```python
from build123d import *

# Parameters (mm, degrees)
F1_DEPTH = 0.26


with BuildPart() as f1:
    # F0 (on Top) → F1 (new body)
    with BuildSketch(Plane.XY):
        with BuildLine():
            ThreePointArc((6.5, 0), (6.4967926424, 0.204169934), (6.4871737348, 0.4081383769))
            ThreePointArc((6.4871737348, 0.4081383769), (6.3848671297, 1.2179785448), (6.1818673559, 2.0086104634))
            ThreePointArc((6.1818673559, 2.0086104634), (5.881375841, 2.7675653952), (5.4881315158, 3.4828741674))
            ThreePointArc((5.4881315158, 3.4828741674), (5.008336078, 4.1432559334), (4.4495561885, 4.7382960782))
            ThreePointArc((4.4495561885, 4.7382960782), (3.8206041399, 5.2586104634), (3.1313988817, 5.6959934203))
            ThreePointArc((3.1313988817, 5.6959934203), (2.3928095925, 6.0435471583), (1.6164842666, 6.2957905473))
            ThreePointArc((1.6164842666, 6.2957905473), (0.8146660182, 6.4487455585), (0, 6.5))
            ThreePointArc((0, 6.5), (-0.8146660182, 6.4487455585), (-1.6164842666, 6.2957905473))
            ThreePointArc((-1.6164842666, 6.2957905473), (-2.3928095925, 6.0435471583), (-3.1313988817, 5.6959934203))
            ThreePointArc((-3.1313988817, 5.6959934203), (-3.8206041399, 5.2586104634), (-4.4495561885, 4.7382960782))
            ThreePointArc((-4.4495561885, 4.7382960782), (-5.008336078, 4.1432559334), (-5.4881315158, 3.4828741674))
            ThreePointArc((-5.4881315158, 3.4828741674), (-5.881375841, 2.7675653952), (-6.1818673559, 2.0086104634))
            ThreePointArc((-6.1818673559, 2.0086104634), (-6.3848671297, 1.2179785448), (-6.4871737348, 0.4081383769))
            ThreePointArc((-6.4871737348, 0.4081383769), (-6.4871737348, -0.4081383769), (-6.3848671297, -1.2179785448))
            ThreePointArc((-6.3848671297, -1.2179785448), (-6.1818673559, -2.0086104634), (-5.881375841, -2.7675653952))
            ThreePointArc((-5.881375841, -2.7675653952), (-5.4881315158, -3.4828741674), (-5.008336078, -4.1432559334))
            ThreePointArc((-5.008336078, -4.1432559334), (-4.4495561885, -4.7382960782), (-3.8206041399, -5.2586104634))
            ThreePointArc((-3.8206041399, -5.2586104634), (-3.1313988817, -5.6959934203), (-2.3928095925, -6.0435471583))
            ThreePointArc((-2.3928095925, -6.0435471583), (-1.6164842666, -6.2957905473), (-0.8146660182, -6.4487455585))
            ThreePointArc((-0.8146660182, -6.4487455585), (0, -6.5), (0.8146660182, -6.4487455585))
            ThreePointArc((0.8146660182, -6.4487455585), (1.6164842666, -6.2957905473), (2.3928095925, -6.0435471583))
            ThreePointArc((2.3928095925, -6.0435471583), (3.1313988817, -5.6959934203), (3.8206041399, -5.2586104634))
            ThreePointArc((3.8206041399, -5.2586104634), (4.4495561885, -4.7382960782), (5.008336078, -4.1432559334))
            ThreePointArc((5.008336078, -4.1432559334), (5.4881315158, -3.4828741674), (5.881375841, -2.7675653952))
            ThreePointArc((5.881375841, -2.7675653952), (6.1818673559, -2.0086104634), (6.3848671297, -1.2179785448))
            ThreePointArc((6.3848671297, -1.2179785448), (6.4711527699, -0.6117040366), (6.5, 0))
        make_face()
    extrude(amount=F1_DEPTH)


solid = f1.part
```
Check sheet for the modelled part. Datum: model origin and axes. Units: mm. Round coordinates to 2 decimals unless told otherwise and drop trailing zeros. Loops run counter-clockwise (first coordinate to the right, second up) from the corner with the lowest first, then second, coordinate; pieces in that order, holes last. Notation, with made-up numbers: (74, 13.5) -> (131, 13.5) arc R23 cw to (131, 51.5) -> close; hole circle Ø3 at (1, -16.5). An arc over 180 degrees is marked (long way). Answer in a Markdown table with one row per item.
Q1. Thickness scan on L1, parallel to X at y = 2, z = 0.1; L2, parallel to X at y = -5.5, z = 0.1; L3, parallel to Y at x = 4.5, z = 0.2. Record the ranges inside material, lowest first.
Data:
| item | result |
|---|---|
| L1 | x = -6.18 to 6.18 |
| L2 | x = -3.46 to 3.46 |
| L3 | y = -4.69 to 4.69 |
Q2. Sectioned sample at B-B on y = -2. Enter the section's corners in (x, z).
Data:
| item | result |
|---|---|
| outline | (-6.18, 0) -> (6.18, 0) -> (6.18, 0.26) -> (-6.18, 0.26) -> close |
Q3. Sectioned sample at A-A on z = 0.05. Enter the section's corners in (x, y).
Data:
| item | result |
|---|---|
| outline | circle Ø13 at (0, 0) |
